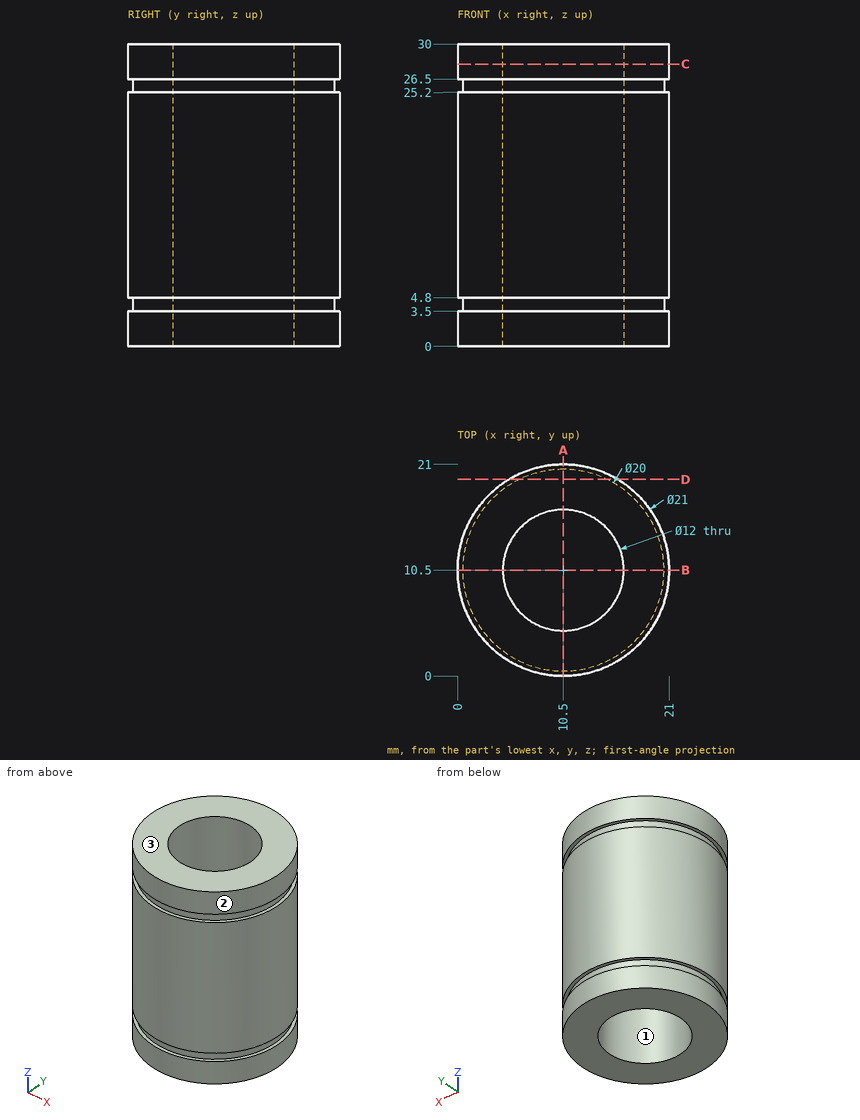
Geometry check sheet. Reference: drawing and pictorial views, mm from the part's lowest x, y, z. Give positions to 0.01 mm unless a question says otherwise; leave off trailing zeros. Order: outer loops, then holes, each group sorted by start corner. A loop starts at its lowest first (then second) coordinate and runs counter-clockwise, first axis right, second up.
1. Release check for a two-part mould opening along X. For the marked faces 1, 2 and 3 record: pulls with the +X half, pulls with the -X half, needs draft (parallel to the pull), parting line crosses it, or undercut.
2. Gauge pin test, flat ends, axial feed: pin 1 Ø6 at (y, z) = (3.5, 26) entering from +X; pin 2 Ø4 at (y, z) = (3.5, 21) entering from -X; pin 3 Ø1 at (y, z) = (7.5, 3.5) entering from -X. Record the tip position at first contact, or that the pin passes through.
3. Section check D-D, the plane y = 19.5. Enter the section's corners in (x, z).
4. Thickness scan on L1, parallel to Y at x = 10.5, z = 27.5; L2, parallel to Y at x = 7.75, z = 5.5; L3, parallel to X at y = 16, z = 25.5. Record the ranges inside material, lowest first.
5. Section check C-C, the plane z = 28. Enter the section's corners in (x, y).
6. Section check A-A, the plane x = 10.5. Enter the section's corners in (y, z), and give its area (3 significant figures).
Values follow:
1. face 1: undercut
1. face 2: parting line crosses it
1. face 3: needs draft
2. pin 1: stops at x = 20.19
2. pin 2: stops at x = 1.27
2. pin 3: stops at x = 0.3
3. outline: (5.09, 0) - (15.91, 0) - (15.91, 3.5) - (14.86, 3.5) - (14.86, 4.8) - (15.91, 4.8) - (15.91, 25.2) - (14.86, 25.2) - (14.86, 26.5) - (15.91, 26.5) - (15.91, 30) - (5.09, 30) - (5.09, 26.5) - (6.14, 26.5) - (6.14, 25.2) - (5.09, 25.2) - (5.09, 4.8) - (6.14, 4.8) - (6.14, 3.5) - (5.09, 3.5) - close
4. L1: y = 0 to 4.5, 16.5 to 21
4. L2: y = 0.37 to 5.17, 15.83 to 20.63
4. L3: x = 2.15 to 8.1, 12.9 to 18.85
5. outline: circle Ø21 at (10.5, 10.5); hole circle Ø12 at (10.5, 10.5)
6. outline: (0, 0) - (4.5, 0) - (4.5, 30) - (0, 30) - (0, 26.5) - (0.5, 26.5) - (0.5, 25.2) - (0, 25.2) - (0, 4.8) - (0.5, 4.8) - (0.5, 3.5) - (0, 3.5) - close; (16.5, 0) - (21, 0) - (21, 3.5) - (20.5, 3.5) - (20.5, 4.8) - (21, 4.8) - (21, 25.2) - (20.5, 25.2) - (20.5, 26.5) - (21, 26.5) - (21, 30) - (16.5, 30) - close
6. area: 267 mm2
